The listing builds one solid part. Answer for the finished solid, in the listing's coordinates (mm). Face numbers are marked on the shaded views. Coordinates: 2 decimals unless noted, no trailing zeros. Write each loop counter-clockwise with the first axis right and the second up, starting at its lowest first coordinate (ties: lowest second). Pieces come first, ordered by that corner, then holes.
from build123d import *

# Parameters (mm, degrees)
F0_W     = 134.9869966507
F0_H     = 47.353733331
F1_DEPTH = 25
F2_SIZE  = 15
F5_D     = 10
F6_D     = 10
F6_DEPTH = 12
F6_TIP   = 3.0043030951
F7_R     = 5


with BuildPart() as f1:
    # F0 (on Top) → F1 (new body)
    with BuildSketch(Plane.XY):
        with Locations((-67.4934983253, -23.6768666655)):
            Rectangle(F0_W, F0_H)
    extrude(amount=F1_DEPTH)

    # F2
    f2_edges = [f1.edges().sort_by_distance(p)[0] for p in [
        (-67.493498, -47.353733, 25),
    ]]
    chamfer(f2_edges, length=F2_SIZE)

    # F5 (through all)
    with Locations(Plane(origin=(0, -28.6768666655, 28.6768666655), x_dir=(1, 0, 0), z_dir=(0, -0.7071067812, 0.7071067812))):
        with Locations((-102.6275157928, -13.9099992812)):
            Hole(F5_D / 2)

    # F6
    with Locations(Plane(origin=(0, -28.6768666655, 28.6768666655), x_dir=(1, 0, 0), z_dir=(0, -0.7071067812, 0.7071067812))):
        with Locations((-51.9247092307, -14.0617964789)):
            Hole(F6_D / 2, depth=F6_DEPTH)
            with Locations((0, 0, -(F6_DEPTH + F6_TIP / 2))):  # 118° drill point
                Cone(0, F6_D / 2, F6_TIP, mode=Mode.SUBTRACT)

    # F7
    f7_edges = [f1.edges().sort_by_distance(p)[0] for p in [
        (0, -23.676867, 0),
    ]]
    fillet(f7_edges, radius=F7_R)


solid = f1.part
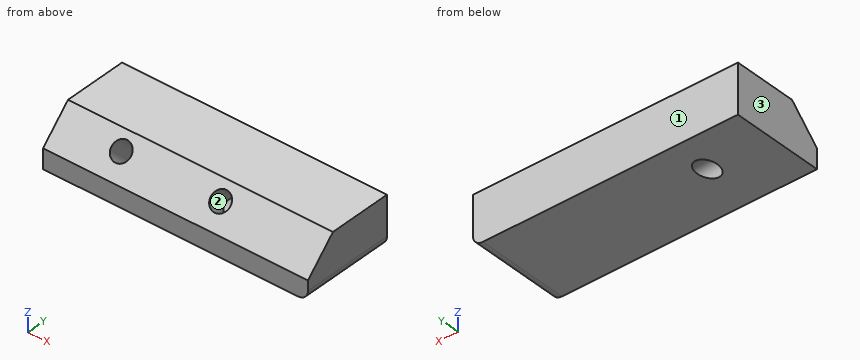
Q1. The part is cut by section B-B, the plane z = 12.25. State how many separate pieces and enclosed holes the cut face has, then the cut area to 3 significant figures.
Answers below:
separate pieces: 1
enclosed holes: 2
area: 5,880 mm2
Q2. Given pin 1 (6 mm diameter, centred on x = -97.5, z = 16, fed in from -Y); pin 2 (5 mm diameter, centred on x = -114.5, z = 18, fed in from -Y), each flat-ended and moving along its own axis, determine where each tip first touches the part or whether it passes through.
Answers below:
pin 1: stops at y = -44.35
pin 2: stops at y = -41.85
Q3. Determine the mould class of the marked faces 1, 2 and 3 for opening direction Y: released by +Y, released by -Y, zero draft, split by the parting line, or undercut.
Answers below:
face 1: released by +Y
face 2: undercut
face 3: zero draft
Q4. The part is cut by section A-A, the plane x = -120. Write down the section's boundary in (y, z).
Answers below:
outline: (-47.35, 0) - (0, 0) - (0, 25) - (-32.35, 25) - (-47.35, 10) - close
Q5. Find the intervals of material crossed by probe 1 along X at (y, z) = (-32, 8.25); probe 2 along Y at (x, z) = (-50.5, 10.25); probe 3 along Y at (x, z) = (-93.5, 18.25), in increasing order.
Answers below:
probe 1: x = -134.99 to -106.71, -98.54 to -55.92, -47.93 to 0
probe 2: y = -47.1 to -36.91, -27.76 to 0
probe 3: y = -39.1 to 0
